Model file for the job. Use its own axes, mm. A direction names the side the tool comes from. Coordinates: 2 decimals unless noted, no trailing zeros. Write each loop counter-clockwise with the first axis right and the second up, starting at its lowest first coordinate (ties: lowest second). Pieces come first, ordered by that corner, then holes. Notation, with made-up numbers: M -9,16 L 11,16 A33 ccw 11,53 Z; hole C -23,-14 d10. An arc over 180 degrees is marked long. Answer in a Markdown table with one row per item. Add a question column.
```python
from build123d import *

# Parameters (mm, degrees)
F0_R     = 1.5
F0_W     = 40.193852
F0_H     = 42.670768
F1_DEPTH = 3.175


with BuildPart() as f1:
    # F0 (on Top) → F1 (new body)
    with BuildSketch(Plane.XY):
        Polygon((-22.673526, -38.870958), (22.326474, -39.071328), (45, -0.20037), (22.673526, 38.870958), (-22.326474, 39.071328), (-45, 0.20037), align=None)
        with Locations((-25, -25)):
            Circle(F0_R, mode=Mode.SUBTRACT)
        with Locations((-0.063241, -28.483691)):
            Circle(F0_R, mode=Mode.SUBTRACT)
        with Locations((-24.69922, -14.187078)):
            Circle(F0_R, mode=Mode.SUBTRACT)
        with Locations((25, -25)):
            Circle(F0_R, mode=Mode.SUBTRACT)
        with Locations((24.63598, -14.296613)):
            Circle(F0_R, mode=Mode.SUBTRACT)
        with Locations((-24.63598, 14.296613)):
            Circle(F0_R, mode=Mode.SUBTRACT)
        with Locations((-25, 25)):
            Circle(F0_R, mode=Mode.SUBTRACT)
        Rectangle(F0_W, F0_H, mode=Mode.SUBTRACT)
        with Locations((24.69922, 14.187078)):
            Circle(F0_R, mode=Mode.SUBTRACT)
        with Locations((0.063241, 28.483691)):
            Circle(F0_R, mode=Mode.SUBTRACT)
        with Locations((25, 25)):
            Circle(F0_R, mode=Mode.SUBTRACT)
    extrude(amount=F1_DEPTH)


solid = f1.part
```
1) Slice it at A-A (x = -25). Give the cut face in (y, z) (3 decimals), then the cut area to 3 significant figures.
2) Drill centre lines: probe 1 along Y at (x, z) = (-0.5, 0.45); probe 2 along Y at (x, z) = (-25, 1.5); probe 3 along X at (y, z) = (-14, 1.8). Where is each one in solid material? Low to high.
3) Two-plate mould, pull along X, no slides. Class faces 3 (the face through (-0.26, 27.02, 1.57)), 4 (the face through (-21, 1, 0)), 5 (the face through (-33.505, 19.908, 1.565)), 6 (the face through (-26.198, -14.121, 1.565)): released by +X, released by -X, zero draft, split by the parting line, or undercut.
4) Flat gauge pins, fed straight in: pin 1 Ø1.5 at (x, z) = (33.5, 0.5) entering from -Y; pin 2 Ø1.5 at (x, z) = (-7.5, 0.5) entering from +Y; pin 3 Ø1.6 at (y, z) = (3.5, 2) entering from +X. Where does each tip first touch, or does it go through?
5) Slice it at D-D (y = -19.5). Give the cut face in (x, z) (3 decimals).
6) Slice it at C-C (z = 0.65). Count the separate pieces of the cut face and the enclosed holes in it, then the cut area to 3 significant figures.
7) Slice it at B-B (y = 25). Give the cut face in (x, z) (3 decimals).
8) Which spindle directions (+Z, -Z, +X, -X, +Y, -Y) get a long thin tool onto all of the face, cutting with end or side? Do faces 1 (the face through (20.097, 0, 2)), 2 (the face through (-21, 1, 3.175)). Say none if no direction does.
Ans:
| question | item | result |
|---|---|---|
| 1 | outline | M -34.8,0 L -26.5,0 L -26.5,3.175 L -34.8,3.175 Z; M -23.5,0 L -15.657,0 L -15.657,3.175 L -23.5,3.175 Z; M -12.718,0 L 12.841,0 L 12.841,3.175 L -12.718,3.175 Z; M 15.752,0 L 23.5,0 L 23.5,3.175 L 15.752,3.175 Z; M 26.5,0 L 34.488,0 L 34.488,3.175 L 26.5,3.175 Z |
| 1 | area | 182 mm2 |
| 2 | probe 1 | y = -38.97 to -29.92, -27.05 to -21.34, 21.34 to 27.09, 29.87 to 38.97 |
| 2 | probe 2 | y = -34.8 to -26.5, -23.5 to -15.66, -12.72 to 12.84, 15.75 to 23.5, 26.5 to 34.49 |
| 2 | probe 3 | x = -36.89 to -26.19, -23.21 to -20.1, 20.1 to 23.17, 26.11 to 36.95 |
| 3 | face 3 | undercut |
| 3 | face 4 | zero draft |
| 3 | face 5 | released by -X |
| 3 | face 6 | undercut |
| 4 | pin 1 | stops at y = -21.2 |
| 4 | pin 2 | stops at y = 39.01 |
| 4 | pin 3 | stops at x = 43.34 |
| 5 | outline | M -33.743,0 L -20.097,0 L -20.097,3.175 L -33.743,3.175 Z; M 20.097,0 L 33.742,0 L 33.742,3.175 L 20.097,3.175 Z |
| 6 | separate pieces | 1 |
| 6 | enclosed holes | 11 |
| 6 | area | 3,480 mm2 |
| 7 | outline | M -30.534,0 L -26.5,0 L -26.5,3.175 L -30.534,3.175 Z; M -23.5,0 L 23.5,0 L 23.5,3.175 L -23.5,3.175 Z; M 26.5,0 L 30.6,0 L 30.6,3.175 L 26.5,3.175 Z |
| 8 | face 1 | +Z, -Z |
| 8 | face 2 | +Z, +X, -X, +Y, -Y |
